Geometry check sheet. Reference: the model listing, model coordinates, mm. Coordinates: 2 decimals unless noted, no trailing zeros. Write each loop counter-clockwise with the first axis right and the second up, starting at its lowest first coordinate (ties: lowest second). Pieces come first, ordered by that corner, then holes. Notation, with made-up numbers: (-36.5, -38.5) -> (-27.5, -38.5) arc R10 cw to (-27.5, -25.5) -> close; hole circle Ø2 at (36.25, 27). An arc over 180 degrees is marked (long way). Answer as CSV lines item,"result".
Autodesk Inventor part; units mm, degrees
ref_plane "YZ Plane" through (0, 0, 0) normal (1, 0, 0) x (0, 1, 0)
ref_plane "XZ Plane" through (0, 0, 0) normal (0, 1, 0) x (-1, 0, 0)
ref_plane "XY Plane" through (0, 0, 0) normal (0, 0, 1) x (1, 0, 0)
sketch "Sketch1" plane through (0, 0, 0) normal (0, 1, 0) x (-1, 0, 0)
  line L0 (17.1429, -30) -> (-22.8571, -30)
  line L1 (-22.8571, -30) -> (-22.8571, -80)
  line L2 (-22.8571, -80) -> (17.1429, -80)
  line L3 (17.1429, -80) -> (17.1429, -30)
  point P0 (0, 0)
  dimension "d0" = 40
  dimension "d1" = 50
extrude "Extrusion1" add sketch "Sketch1" along normal blind 10.475
sketch "Sketch3" plane through (22.8571, 0, -80) normal (0, 0, -1) x (-1, 0, 0)
  line L0 (0, 0) -> (40, 0)
  line L1 (0, 10.475) -> (40, 10.475)
  line L2 (40, 10.475) -> (40, 0)
  line L3 (40, 0) -> (0, 0)
  line L4 (0, 0) -> (0, 10.475)
  point P0 (22.8571, 0)
extrude "Extrusion3" add sketch "Sketch3" along normal blind 11.252
full round fillet "Fillet1" first side at (9.5238, 10.475, -50.4173) centre faces at (9.5238, 3.4917, -91.252) second side at (9.5238, 0, -70.8347)
sketch "Sketch6" plane through (0, 0, 0) normal (0, -1, 0) x (1, 0, 0)
  line L0 (22.8571, -30) -> (22.8571, -86.0145)
  line L1 (-17.1429, -91.252) -> (-17.1429, -86.0145)
  line L2 (22.8571, -30) -> (-17.1429, -30)
  line L3 (-17.1429, -30) -> (-17.1429, -91.252)
  line L4 (-17.1429, -91.252) -> (22.8571, -91.252)
  line L5 (22.8571, -91.252) -> (22.8571, -30)
  point P0 (0, 0)
extrude "Extrusion5" cut sketch "Sketch6" against normal blind 10.7
ref_plane "Work Plane5" through (0, 10.475, 0) normal (0, -1, 0) x (1, 0, 0)
sketch "Sketch8" plane through (0, 10.475, 0) normal (0, -1, 0) x (1, 0, 0)
  line L0 (-0.1429, -97) -> (-0.1429, -83)
  line L1 (-0.1429, -91.5044) -> (22.8571, -91.5044)
  line L2 (22.8571, -91.5044) -> (22.8571, -141.5044)
  line L3 (22.8571, -141.5044) -> (-0.1429, -141.5044)
  line L4 (-0.1429, -141.5044) -> (-0.1429, -91.5044)
  line L5 (-0.1429, -91.5044) -> (-17.1429, -91.5044)
  line L6 (-17.1429, -91.5044) -> (-17.1429, -141.5044)
  line L7 (-17.1429, -141.5044) -> (-0.1429, -141.5044)
  line L8 (-0.1429, -141.5044) -> (-0.1429, -91.5044)
  point P0 (0, 0)
  dimension "d14" = 23
  dimension "d15" = 50
  dimension "d16" = 17
extrude "Extrusion6" add sketch "Sketch8" along normal blind 10.7
full round fillet "Fillet2" first side at (15.1905, 10.475, -124.8377) centre faces at (15.1905, 6.9083, -91.5044) second side at (15.1905, -0.225, -124.8377)
sketch "Sketch9" plane through (-17.1429, -0.225, -141.5044) normal (-1, 0, 0) x (0, 0, 1)
  line L0 (0, 10.7) -> (44.65, 10.7)
  line L1 (0, 10.7) -> (0, 0)
  line L2 (44.65, 10.7) -> (0, 0)
  line L3 (0, 0) -> (0, 10.7)
  arc A0 (44.65, 0) -> (44.65, 10.7) centre (44.65, 5.35) ccw
  line L4 (0, 10.7) -> (44.65, 10.7)
  point P0 (141.5044, 0.225)
extrude "Extrusion7" cut sketch "Sketch9" against normal blind 40
sketch "Sketch10" plane through (-17.1429, 5.125, -96.8544) normal (-1, 0, 0) x (0, 0, 1)
  line L0 (0, -1) -> (-0.866, -0.5)
  line L1 (-0.866, -0.5) -> (-0.866, 0.5)
  line L2 (-0.866, 0.5) -> (0, 1)
  line L3 (0, 1) -> (0.866, 0.5)
  line L4 (0.866, 0.5) -> (0.866, -0.5)
  line L5 (0.866, -0.5) -> (0, -1)
  point P0 (96.8544, -5.125)
  point P1 (0, 0)
extrude "Extrusion8" add sketch "Sketch10" along normal blind 2
sketch "Sketch11" plane through (22.8571, 5.125, -96.8544) normal (1, 0, 0) x (0, 0, -1)
  line L0 (0, -1) -> (-0.866, -0.5)
  line L1 (0, -1) -> (-0.866, -0.5)
  line L2 (-0.866, -0.5) -> (-0.866, 0.5)
  line L3 (-0.866, 0.5) -> (0, 1)
  line L4 (0, 1) -> (0.866, 0.5)
  line L5 (0.866, 0.5) -> (0.866, -0.5)
  line L6 (0.866, -0.5) -> (0, -1)
  point P0 (-96.8544, -5.125)
  point P1 (0, 0)
extrude "Extrusion9" add sketch "Sketch11" along normal blind 2
Item 1: Cross-section at B-B, the plane z = -120. Record the cut outline in (x, y) (3 decimals).
Responses:
outline,"(-17.143, -0.225) -> (22.857, -0.225) -> (22.857, 4.928) -> (-17.143, 4.928) -> close"
Item 2: Cross-section at C-C, the plane y = 8. Record the cut outline in (x, z), plus the area to 3 significant figures.
Responses:
outline,"(-17.14, -107.18) -> (22.86, -107.18) -> (22.86, -92.34) -> (-17.14, -92.34) -> close"
area,"594 mm2"
Item 3: Depth check by flat-ended pin: pin 1 Ø1.5 at (y, z) = (9, -101) entering from -X; pin 2 Ø0.8 at (x, y) = (23.5, 5.5) entering from +Z; pin 3 Ø1.5 at (y, z) = (4.5, -133.5) entering from +X; pin 4 Ø0.8 at (x, y) = (-18.5, 5) entering from -Z. Enter the tip coordinate at first touch or a pass-through.
Responses:
pin 1,"stops at x = -17.14"
pin 2,"stops at z = -95.99"
pin 3,"passes through"
pin 4,"stops at z = -97.72"
Item 4: Thickness scan on probe 1 along X at (y, z) = (2.25, -117); probe 2 along Y at (x, z) = (17, -115) (3 decimals); probe 3 along Y at (x, z) = (-14.5, -132) (3 decimals). Record the ranges inside material, lowest first.
Responses:
probe 1,"x = -17.14 to 22.86"
probe 2,"y = -0.225 to 6.127"
probe 3,"y = -0.225 to 2.053"
